Geometry: see drawing. Coordinates: mm, zero at the bounding-box minimum. Round coordinates to 2 decimals unless told otherwise and drop trailing zeros. Loops run counter-clockwise (first coordinate to the right, second up) from the corner with the lowest first, then second, coordinate; pieces in that order, holes last. Notation, with made-up numbers: (45, 33) - (55, 33) arc R28 cw to (55, 62) - close; hole circle Ø2 at (-11.5, 40.25). An arc over 180 degrees is marked (long way). Answer in a Markdown table with one row per item. Add a question column.
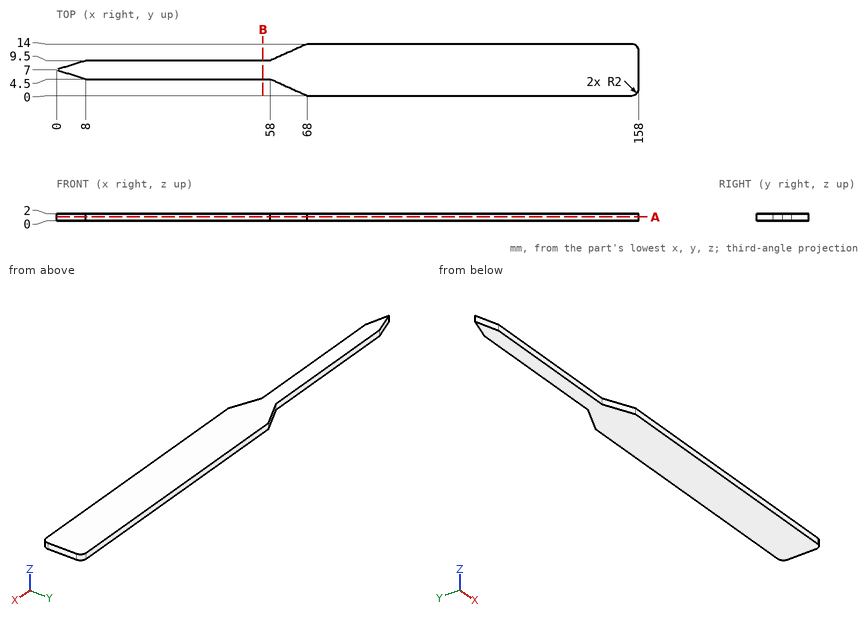
1) Section B-B, the plane x = 56. Return the cut outline in (y, z).
2) Material intervals for line 1 along Y through (x, z) = (54, 1.35); line 2 along X through (y, z) = (3.5, 1.15); line 3 along X through (y, z) = (12.25, 0.25), sorted ascending. Write a range as from..to.
3) Contact query for flat-ended pins moving along their axis: pin 1 Ø0.6 at (x, z) = (21, 1.5) entering from -Y; pin 2 Ø1 at (x, z) = (39, 1.5) entering from +Y. Output: stop coordinate, or through.
4) Section A-A, the plane z = 1.1. Return the cut outline in (x, y), and give its area (3 significant figures).
Evaluation:
| question | item | result |
|---|---|---|
| 1 | outline | (4.5, 0) - (9.5, 0) - (9.5, 2) - (4.5, 2) - close |
| 2 | line 1 | y = 4.5..9.5 |
| 2 | line 2 | x = 60.22..158 |
| 2 | line 3 | x = 64.11..157.98 |
| 3 | pin 1 | stops at y = 4.5 |
| 3 | pin 2 | stops at y = 9.5 |
| 4 | outline | (0, 7) - (8, 4.5) - (58, 4.5) - (68, 0) - (156, 0) arc R2 ccw to (158, 2) - (158, 12) arc R2 ccw to (156, 14) - (68, 14) - (58, 9.5) - (8, 9.5) - close |
| 4 | area | 1,620 mm² |
